Geometry: final body of the model. Coordinates: model frame, mm. Face numbers are marked on the shaded views. A direction names the side the tool comes from. Round coordinates to 2 decimals unless told otherwise and drop trailing zeros. Loops run counter-clockwise (first coordinate to the right, second up) from the corner with the lowest first, then second, coordinate; pieces in that order, holes last. Notation, with made-up numbers: (72, -35.5) - (105, -35.5) arc R35 ccw to (105, -0.5) - close; hole circle Ø8 at (73.25, -19.5). An arc over 180 degrees is marked (long way). Return JSON: item names as keys, results as strings. Group by question number.
1. First-contact query: pin 1 Ø1.4 at (x, y) = (-28, -5.5) entering from +Z; pin 2 Ø6.5 at (x, y) = (0, 14) entering from -Z; pin 3 Ø14.5 at (x, z) = (18.5, 7.5) entering from +Y; pin 4 Ø5 at (y, z) = (-5, -2) entering from -X. Flat tips, straight axial feed; report the tip coordinate or a pass-through.
2. Material intervals for probe 1 along Y at (x, z) = (-20, 5.5); probe 2 along Z at (x, y) = (-29, -10.8); probe 3 along X at (y, z) = (-9.85, 0), sorted ascending.
3. Section B-B on y = -19. Return loops of the section in (x, z), and give its area (3 significant figures).
4. Section C-C on x = 0. Return loops of the section in (y, z), and give its area (3 significant figures).
5. Section A-A on z = 0. Return loops of the section in (x, y), and give its area (3 significant figures).
6. Section D-D on z = -13. Return loops of the section in (x, y), and give its area (3 significant figures).
7. Draft query along Z for the marked faces 1, 2, 3 and 4. Return one class per face: +Z half, -Z half, draft (parallel to the pull), parting line (faces both ways), or undercut.
8. Set-up query: the marked faces 5, 6, 7 and 8. Return all of +Z, -Z, +X, -X, +Y, -Y with unobstructed straight access to the full face (end or side cutting, diameter ignored); none if empty.
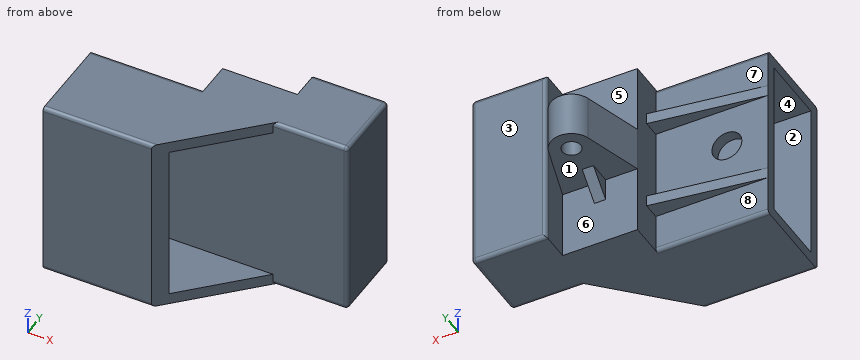
from build123d import *

# Parameters (mm, degrees)
EXTRUDE_1_DEPTH         = 30
EXTRUDE_1_DEPTH_BACK    = 40
SKETCH_2_W              = 49
SKETCH_2_H              = 24
SKETCH_2_W_2            = 43
SKETCH_2_H_2            = 18
SKETCH_1_R              = 2.5
EXTRUDE_1_2_DEPTH       = 6
SKETCH_1_3_W            = 20
SKETCH_1_3_H            = 8
EXTRUDE_2_DEPTH         = 24.5
CUT_EXTRUDE_1_DEPTH     = 25
RIB_1_REACH             = 58.032
SKETCH_4_WALLS_W        = 145.49538697
SKETCH_4_WALLS_H        = 3
RIB_2_REACH             = 65.649
SKETCH_6_WALLS_W        = 3
SKETCH_6_WALLS_H        = 137.784142328
CUT_EXTRUDE_START       = -12
CUT_EXTRUDE_2_OUTLINE_R = 4
CUT_EXTRUDE_2_DEPTH     = 3
FILLET_1_R              = 1


# Read off the part's stored shape, not the designer's step: the extrude step
with BuildPart() as part:
    # Sketch 2 → Extrude 1 (new, two sides: drawn at the far end of the back side and taken through both)
    with BuildSketch(Plane(origin=(0, 0, 0), x_dir=(0, 0, -1), z_dir=(1, 0, 0)).offset(-EXTRUDE_1_DEPTH_BACK)):
        with Locations((0, -21)):
            Rectangle(SKETCH_2_W, SKETCH_2_H)
        with Locations((0, -21)):
            Rectangle(SKETCH_2_W_2, SKETCH_2_H_2, mode=Mode.SUBTRACT)
    extrude(amount=EXTRUDE_1_DEPTH + EXTRUDE_1_DEPTH_BACK)



with BuildPart() as body_2:
    # Sketch 1 → Extrude 1 2 (new, symmetric)
    with BuildSketch(Plane.XY):
        with BuildLine():
            ThreePointArc((-5.262640911, 15.598314937), (0, 19.5), (5.262640911, 15.598314937))
            Line((5.262640911, 15.598314937), (10, 0))
            Line((10, 0), (-10, 0))
            Line((-10, 0), (-5.262640911, 15.598314937))
        make_face()
        with Locations((0, 14)):
            Circle(SKETCH_1_R, mode=Mode.SUBTRACT)
    extrude(amount=EXTRUDE_1_2_DEPTH, both=True)


with BuildPart() as part_1:
    add(part.part)

    add(body_2.part)  # Extrude 2 merges body 2
    # Sketch 1_3 → Extrude 2 (add, symmetric)
    with BuildSketch(Plane.XY):
        Polygon((10, 0), (-10, 0), (-10, -12), (10, -12), (30, -12), (30, 0), align=None)
        with Locations((20, 4)):
            Rectangle(SKETCH_1_3_W, SKETCH_1_3_H)
    extrude(amount=EXTRUDE_2_DEPTH, both=True)

    # Sketch 1_4 → Cut-Extrude 1 (cut, symmetric)
    with BuildSketch(Plane.XY):
        Polygon((30, -12), (10, -12), (-11, -33), (30, -33), align=None)
    extrude(amount=CUT_EXTRUDE_1_DEPTH, both=True, mode=Mode.SUBTRACT)

    # Sketch 4 walls → Rib 1 (add, up to next)
    with BuildSketch(Plane(origin=(0.4400978, -2.93398533, 0), x_dir=(0.9889363528682976, 0.14834045293024456, 0), z_dir=(-0.14834045293024456, 0.9889363528682976, 0)), mode=Mode.PRIVATE) as rib_1_sk1:
        with Locations((-25.177107795, -12.5)):
            Rectangle(SKETCH_4_WALLS_W, SKETCH_4_WALLS_H)
    rib_1_tool1 = extrude(rib_1_sk1.sketch, amount=-RIB_1_REACH, mode=Mode.PRIVATE) - part_1.part
    # Sketch 4 walls → Rib 1 (add, up to next)
    with BuildSketch(Plane(origin=(0.4400978, -2.93398533, 0), x_dir=(0.9889363528682976, 0.14834045293024456, 0), z_dir=(-0.14834045293024456, 0.9889363528682976, 0)), mode=Mode.PRIVATE) as rib_1_sk2:
        with Locations((-25.177107795, 12.5)):
            Rectangle(SKETCH_4_WALLS_W, SKETCH_4_WALLS_H)
    rib_1_tool2 = extrude(rib_1_sk2.sketch, amount=-RIB_1_REACH, mode=Mode.PRIVATE) - part_1.part
    add(rib_1_tool1.solids().sort_by_distance((-24.458459359, -6.668768904, 12.5))[0])
    add(rib_1_tool2.solids().sort_by_distance((-24.458459359, -6.668768904, -12.5))[0])

    # Sketch 6 walls → Rib 2 (add, up to next)
    with BuildSketch(Plane(origin=(0, 6, -6), x_dir=(1, 0, 0), z_dir=(0, 0.7071067811865477, -0.7071067811865474)), mode=Mode.PRIVATE) as rib_2_sk1:
        with Locations((0, 4.242640687)):
            Rectangle(SKETCH_6_WALLS_W, SKETCH_6_WALLS_H)
    rib_2_tool1 = extrude(rib_2_sk1.sketch, amount=-RIB_2_REACH, mode=Mode.PRIVATE) - part_1.part
    rib_2 = rib_2_tool1.solids().sort_by_distance((0, 3, -9))[0]
    add(rib_2)

    # Mirror 1: Rib 2 across plane
    add(rib_2.mirror(Plane.XY))

    # Cut-Extrude 2 outline → Cut-Extrude 2 (cut)
    with BuildSketch(Plane(origin=(0, 0, 0), x_dir=(1, 0, 0), z_dir=(0, 1, 0)).offset(CUT_EXTRUDE_START)):
        with Locations((-29, 0)):
            Circle(CUT_EXTRUDE_2_OUTLINE_R)
    extrude(amount=CUT_EXTRUDE_2_DEPTH, mode=Mode.SUBTRACT)

    # Fillet 1
    fillet_1_edges = [part_1.edges().sort_by_distance(p)[0] for p in [
        (30, -2, 24.5),
        (30, -12, 0),
        (20, 8, -24.5),
        (30, 8, 0),
        (10, 8, 0),
        (20, 8, 24.5),
        (-25.5, -33, 24.5),
        (-25, -9, 24.5),
        (-25, -9, -24.5),
        (-25.5, -33, -24.5),
        (30, -2, -24.5),
        (20, -12, 24.5),
        (20, -12, -24.5),
    ]]
    fillet(fillet_1_edges, radius=FILLET_1_R)


solid = part_1.part
Taken from the geometry:
{
 "1": {"pin 1": "through", "pin 2": "z = -6", "pin 3": "y = 8", "pin 4": "x = -10"},
 "2": {"probe 1": "-33 to -30, -12 to -9", "probe 2": "-24.5 to -4, 4 to 24.5", "probe 3": "-40 to -33, -25 to 30"},
 "3": {"outline": "(-40, -24.5) - (3, -24.5) - (3, -21.5) - (-40, -21.5) - close; (-40, 21.5) - (3, 21.5) - (3, 24.5) - (-40, 24.5) - close", "area": "258 mm2"},
 "4": {"outline": "(-22, -24.5) - (0, -24.5) - (0, -12) - (6, -6) - (11.5, -6) - (11.5, 6) - (6, 6) - (0, 12) - (0, 24.5) - (-22, 24.5) - (-22, 21.5) - (-12, 21.5) - (-12, -21.5) - (-22, -21.5) - close; (16.5, -6) - (19.5, -6) - (19.5, 6) - (16.5, 6) - close", "area": "858 mm2"},
 "5": {"outline": "(-40, -33) - (-11, -33) - (-8, -30) - (-40, -30) - close; (-40, -12) - (-33, -12) - (-33, -9) - (-40, -9) - close; (-25, -12) - (29, -12) arc R1 ccw to (30, -11) - (30, 7) arc R1 ccw to (29, 8) - (11, 8) arc R1 ccw to (10, 7) - (10, 0) - (5.26, 15.6) arc R5.5 ccw to (-5.26, 15.6) - (-10, 0) - (-10, -9) - (-25, -9) - close; hole circle Ø5 at (0, 14)", "area": "1,050 mm2"},
 "6": {"outline": "(-40, -33) - (-11, -33) - (-8, -30) - (-40, -30) - close; (-40, -12) - (29, -12) arc R1 ccw to (30, -11) - (30, 7) arc R1 ccw to (29, 8) - (11, 8) arc R1 ccw to (10, 7) - (10, 0) - (-10, 0) - (-10, -4.5) - (-40, -9) - close", "area": "888 mm2"},
 "7": {"face 1": "-Z half", "face 2": "undercut", "face 3": "draft", "face 4": "undercut"},
 "8": {"face 5": "+Z, +Y", "face 6": "-Z, +Y", "face 7": "+Z, -X, +Y", "face 8": "-Z, -X, +Y"}
}
